Work out the finished part from the listing and answer in its coordinate system (mm). Coordinates: 2 decimals unless noted, no trailing zeros. Order: outer loops, then holes, each group sorted by start corner. A loop starts at its lowest first (then second) coordinate and runs counter-clockwise, first axis right, second up. Notation, with made-up numbers: M 74,81 L 113,81 A12 cw 113,91 Z; hole C -2.75,58 d10. An arc over 180 degrees is marked long. Write item = value, one per line. Start each with the question number.
Q1. Find section A-A on z = -43. Give the vertices of the cut face in (x, y) (3 decimals).
Q2. Find section B-B on y = 1.55. Give the number of separate pieces and of enclosed holes in the cut face, and give its area (3 significant figures).
Q3. Straight lines are drawn through the part: line 1 along Z through (x, y) = (77.5, 2.6); line 2 along X through (y, z) = (2.25, -28) (3 decimals); line 3 along X through (y, z) = (2.3, -12) (3 decimals). For each, find the intervals that lie inside material, in ascending order.
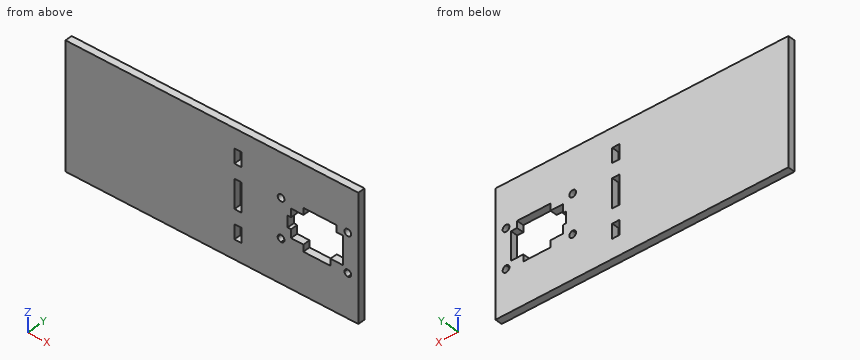
```python
from build123d import *

# Parameters (mm, degrees)
SKETCH1_W           = 130
SKETCH1_H           = 55
SKETCH1_W_2         = 3.175
SKETCH1_H_2         = 6.35
SKETCH1_H_3         = 12.7
BOSS_EXTRUDE1_DEPTH = 3.175


with BuildPart() as part:
    # Sketch1 → Boss-Extrude1 (new body)
    with BuildSketch(Plane(origin=(0, 0, 0), x_dir=(1, 0, 0), z_dir=(0, 1, 0))):
        with Locations((65, 27.5)):
            Rectangle(SKETCH1_W, SKETCH1_H)
        with Locations((76.5875, 43.375)):
            Rectangle(SKETCH1_W_2, SKETCH1_H_2, mode=Mode.SUBTRACT)
        with Locations((76.5875, 11.625)):
            Rectangle(SKETCH1_W_2, SKETCH1_H_2, mode=Mode.SUBTRACT)
        with Locations((76.5875, 27.5)):
            Rectangle(SKETCH1_W_2, SKETCH1_H_3, mode=Mode.SUBTRACT)
        Polygon((98.622387284, 25), (100.122287284, 25), (100.122287284, 21.3), (105.622287284, 21.3), (105.622287284, 18.3002), (120.422287284, 18.3002), (120.422287284, 21.3), (123.122287284, 21.3), (123.122287284, 33.7), (117.622287284, 33.7), (117.622287284, 36.7), (105.622287284, 36.7), (105.622287284, 33.7), (100.122287284, 33.7), (100.122287284, 30), (98.622387284, 30), align=None, mode=Mode.SUBTRACT)
        with BuildLine():
            add(Edge.make_bspline(
                [(97.222287284, 36), (97.222287284, 35.1715), (96.550787284, 34.5), (95.722387284, 34.5)],
                knots=[0, 0, 0, 0, 0.2, 0.2, 0.2, 0.2], degree=3))
            add(Edge.make_bspline(
                [(95.722387284, 34.5), (94.893887284, 34.4999), (94.222387284, 35.1715), (94.222387284, 35.9999)],
                knots=[0.2, 0.2, 0.2, 0.2, 0.4, 0.4, 0.4, 0.4], degree=3))
            add(Edge.make_bspline(
                [(94.222387284, 35.9999), (94.222287284, 36.8284), (94.893887284, 37.4999), (95.722287284, 37.5)],
                knots=[0.4, 0.4, 0.4, 0.4, 0.6, 0.6, 0.6, 0.6], degree=3))
            add(Edge.make_bspline(
                [(95.722287284, 37.5), (96.550787284, 37.5), (97.222287284, 36.8284), (97.222287284, 36)],
                knots=[0.6, 0.6, 0.6, 0.6, 1, 1, 1, 1], degree=3))
        make_face(mode=Mode.SUBTRACT)
        with BuildLine():
            add(Edge.make_bspline(
                [(126.822287284, 19.0002), (126.822287284, 18.1718), (126.150687284, 17.5002), (125.322387284, 17.5002)],
                knots=[0, 0, 0, 0, 0.2, 0.2, 0.2, 0.2], degree=3))
            add(Edge.make_bspline(
                [(125.322387284, 17.5002), (124.493987284, 17.5002), (123.822387284, 18.1718), (123.822387284, 19.0001)],
                knots=[0.2, 0.2, 0.2, 0.2, 0.4, 0.4, 0.4, 0.4], degree=3))
            add(Edge.make_bspline(
                [(123.822387284, 19.0001), (123.822387284, 19.8285), (124.493987284, 20.4999), (125.322287284, 20.4999)],
                knots=[0.4, 0.4, 0.4, 0.4, 0.6, 0.6, 0.6, 0.6], degree=3))
            add(Edge.make_bspline(
                [(125.322287284, 20.4999), (126.150687284, 20.4999), (126.822287284, 19.8285), (126.822287284, 19.0002)],
                knots=[0.6, 0.6, 0.6, 0.6, 1, 1, 1, 1], degree=3))
        make_face(mode=Mode.SUBTRACT)
        with BuildLine():
            add(Edge.make_bspline(
                [(97.222287284, 19.0002), (97.222287284, 18.1718), (96.550687284, 17.5001), (95.722387284, 17.5001)],
                knots=[0, 0, 0, 0, 0.2, 0.2, 0.2, 0.2], degree=3))
            add(Edge.make_bspline(
                [(95.722387284, 17.5001), (94.893987284, 17.5001), (94.222287284, 18.1718), (94.222287284, 19.0001)],
                knots=[0.2, 0.2, 0.2, 0.2, 0.4, 0.4, 0.4, 0.4], degree=3))
            add(Edge.make_bspline(
                [(94.222287284, 19.0001), (94.222287284, 19.8285), (94.893987284, 20.5), (95.722287284, 20.5)],
                knots=[0.4, 0.4, 0.4, 0.4, 0.6, 0.6, 0.6, 0.6], degree=3))
            add(Edge.make_bspline(
                [(95.722287284, 20.5), (96.550687284, 20.5), (97.222287284, 19.8285), (97.222287284, 19.0002)],
                knots=[0.6, 0.6, 0.6, 0.6, 1, 1, 1, 1], degree=3))
        make_face(mode=Mode.SUBTRACT)
        with BuildLine():
            add(Edge.make_bspline(
                [(126.822287284, 36), (126.822287284, 35.1715), (126.150787284, 34.5001), (125.322387284, 34.5001)],
                knots=[0, 0, 0, 0, 0.2, 0.2, 0.2, 0.2], degree=3))
            add(Edge.make_bspline(
                [(125.322387284, 34.5001), (124.493887284, 34.5), (123.822487284, 35.1715), (123.822487284, 35.9999)],
                knots=[0.2, 0.2, 0.2, 0.2, 0.4, 0.4, 0.4, 0.4], degree=3))
            add(Edge.make_bspline(
                [(123.822487284, 35.9999), (123.822387284, 36.8284), (124.493887284, 37.4998), (125.322287284, 37.4999)],
                knots=[0.4, 0.4, 0.4, 0.4, 0.6, 0.6, 0.6, 0.6], degree=3))
            add(Edge.make_bspline(
                [(125.322287284, 37.4999), (126.150787284, 37.4999), (126.822287284, 36.8284), (126.822287284, 36)],
                knots=[0.6, 0.6, 0.6, 0.6, 1, 1, 1, 1], degree=3))
        make_face(mode=Mode.SUBTRACT)
    extrude(amount=BOSS_EXTRUDE1_DEPTH)


solid = part.part
```
Findings below:
q1.outline = M 0,0 L 75,0 L 75,3.175 L 0,3.175 Z; M 78.175,0 L 130,0 L 130,3.175 L 78.175,3.175 Z
q2.separate_pieces = 1
q2.enclosed_holes = 8
q2.area = 6,670 mm^2
q3.line_1 = -55 to -46.55, -40.2 to -33.85, -21.15 to -14.8, -8.45 to 0
q3.line_2 = 0 to 75, 78.175 to 98.622, 123.122 to 130
q3.line_3 = 0 to 75, 78.175 to 130
